The listing builds one solid part. Answer for the finished solid, in the listing's coordinates (mm). Face numbers are marked on the shaded views. A direction names the side the tool comes from. Coordinates: 2 decimals unless noted, no trailing zeros. Order: outer loops, then holes, each group sorted by start corner. A loop starts at its lowest first (then second) coordinate and runs counter-clockwise, first axis right, second up. Notation, with made-up numbers: (60, -4) -> (66, -4) arc R23 ccw to (66, 32) -> close; hole circle Ø1 at (55, 47). An arc over 180 degrees is marked (long way). Return JSON: item names as keys, results as strings.
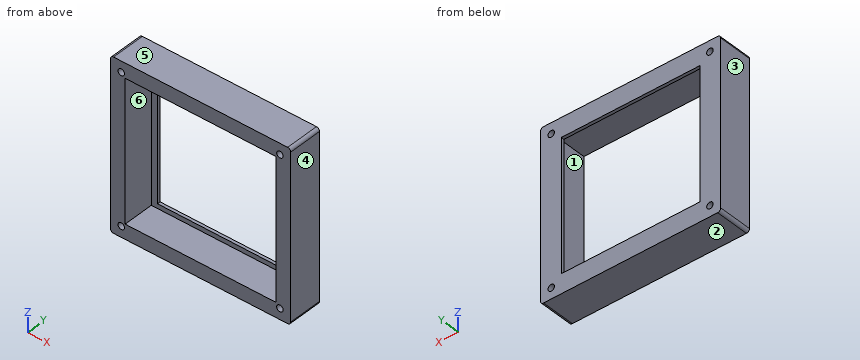
```python
from build123d import *

# Parameters (mm, degrees)
SKETCH009_W     = 58.5
SKETCH009_H     = 55
PAD005_DEPTH    = 11
SKETCH010_W     = 49
SKETCH010_H     = 45.5
POCKET004_DEPTH = 10
SKETCH011_W     = 45
SKETCH011_H     = 42.5
POCKET005_DEPTH = 5
SKETCH012_R     = 1.05
POCKET006_DEPTH = 12
FILLET003_R     = 1


with BuildPart() as part:
    # Sketch009 → Pad005 (new body)
    with BuildSketch(Plane.XZ):
        Rectangle(SKETCH009_W, SKETCH009_H)
    extrude(amount=-PAD005_DEPTH)

    # Sketch010 (on Face5 of Pad005) → Pocket004 (cut)
    with BuildSketch(Plane.XZ):
        Rectangle(SKETCH010_W, SKETCH010_H)
    extrude(amount=-POCKET004_DEPTH, mode=Mode.SUBTRACT)

    # Sketch011 (on Face11 of Pocket004) → Pocket005 (cut)
    with BuildSketch(Plane.XZ.offset(-10)):
        Rectangle(SKETCH011_W, SKETCH011_H)
    extrude(amount=-POCKET005_DEPTH, mode=Mode.SUBTRACT)

    # Sketch012 (on Face4 of Pocket005) → Pocket006 (cut)
    with BuildSketch(Plane.XZ):
        with Locations((-25.75, 24)):
            Circle(SKETCH012_R)
        with Locations((25.75, 24)):
            Circle(SKETCH012_R)
        with Locations((-25.75, -24)):
            Circle(SKETCH012_R)
        with Locations((25.75, -24)):
            Circle(SKETCH012_R)
    extrude(amount=-POCKET006_DEPTH, mode=Mode.SUBTRACT)

    # Fillet003
    fillet003_edges = [part.edges().sort_by_distance(p)[0] for p in [
        (29.25, 5.5, 27.5),
        (29.25, 5.5, -27.5),
        (-29.25, 5.5, 27.5),
        (-29.25, 5.5, -27.5),
    ]]
    fillet(fillet003_edges, radius=FILLET003_R)


solid = part.part
```
Item 1: Find the intervals of material crossed by probe 1 along Z at (x, y) = (25.75, 3.5); probe 2 along X at (y, z) = (9.25, 17.5); probe 3 along Z at (x, y) = (-16.5, 6.75), in increasing order.
Answer list:
{"probe 1": "-27.5 to -25.05, -22.95 to 22.95, 25.05 to 27.5", "probe 2": "-29.25 to -24.5, 24.5 to 29.25", "probe 3": "-27.5 to -22.75, 22.75 to 27.5"}
Item 2: Which of the six approach directions +Z, -Z, +X, -X, +Y, -Y give full straight-line access (tool end or side, diameter ignored) to the marked faces 5 and 6?
Answer list:
{"face 5": "+Z, +X, -X, +Y, -Y", "face 6": "-Y"}
Item 3: A flat-ended cylindrical pin translates along its axis: pin 1 (12 mm diameter, centred on x = -17, z = -7.5, fed in from -Y). Find the tip coordinate at first contact, or state that the pin passes through.
Answer list:
{"pin 1": "y = 10"}
Item 4: The part is cut by section C-C on y = 1. Determine the outline of the cut face in (x, z).
Answer list:
{"outline": "(-29.25, -26.5) arc R1 ccw to (-28.25, -27.5) -> (28.25, -27.5) arc R1 ccw to (29.25, -26.5) -> (29.25, 26.5) arc R1 ccw to (28.25, 27.5) -> (-28.25, 27.5) arc R1 ccw to (-29.25, 26.5) -> close; hole circle Ø2.1 at (-25.75, -24); hole circle Ø2.1 at (-25.75, 24); hole (-24.5, -22.75) -> (24.5, -22.75) -> (24.5, 22.75) -> (-24.5, 22.75) -> close; hole circle Ø2.1 at (25.75, -24); hole circle Ø2.1 at (25.75, 24)"}
Item 5: The part is cut by section A-A on x = 25.75. Determine the outline of the cut face in (y, z).
Answer list:
{"outline": "(0, -27.5) -> (11, -27.5) -> (11, -25.05) -> (0, -25.05) -> close; (0, -22.95) -> (11, -22.95) -> (11, 22.95) -> (0, 22.95) -> close; (0, 25.05) -> (11, 25.05) -> (11, 27.5) -> (0, 27.5) -> close"}
Item 6: The part is cut by section D-D on x = -5.5. Determine the outline of the cut face in (y, z), plus the area to 4 significant figures.
Answer list:
{"outline": "(0, -27.5) -> (11, -27.5) -> (11, -21.25) -> (10, -21.25) -> (10, -22.75) -> (0, -22.75) -> close; (0, 22.75) -> (10, 22.75) -> (10, 21.25) -> (11, 21.25) -> (11, 27.5) -> (0, 27.5) -> close", "area": "107.5 mm2"}
Item 7: The part is cut by section B-B on z = 24. Determine the outline of the cut face in (x, y).
Answer list:
{"outline": "(-29.25, 0) -> (-26.8, 0) -> (-26.8, 11) -> (-29.25, 11) -> close; (-24.7, 0) -> (24.7, 0) -> (24.7, 11) -> (-24.7, 11) -> close; (26.8, 0) -> (29.25, 0) -> (29.25, 11) -> (26.8, 11) -> close"}
Item 8: Determine the mould class of the marked faces 1, 2, 3 and 4 for opening direction X: pulls with the +X half, pulls with the -X half, needs draft (parallel to the pull), parting line crosses it, or undercut.
Answer list:
{"face 1": "undercut", "face 2": "needs draft", "face 3": "pulls with the -X half", "face 4": "pulls with the +X half"}
